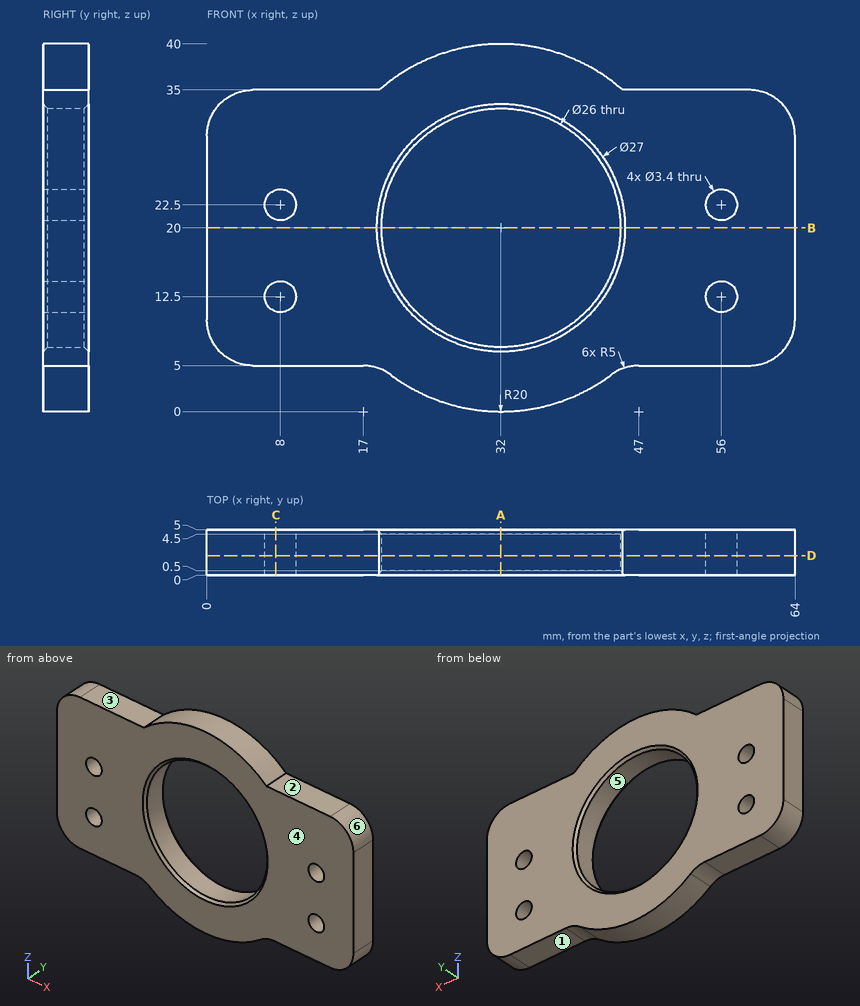
Input: dimensioned drawing with shaded views. Units: mm. Origin: part minimum x, y, z. A direction names the side the tool comes from. Round coordinates to 2 decimals unless told otherwise and drop trailing zeros. Loops run counter-clockwise (first coordinate to the right, second up) from the corner with the lowest first, then second, coordinate; pieces in that order, holes last. Notation, with made-up numbers: (67.5, 89.25) -> (85.5, 89.25) arc R20 cw to (85.5, 94.25) -> close; hole circle Ø10 at (-25, 84.5). An arc over 180 degrees is marked (long way). Answer as a JSON object with one key per item and string values. Group by question number.
Q1. Section query C-C (x = 7.5). Output: boundary loops of the cut face in (y, z).
Q2. Contact query for flat-ended pins moving along their axis: P1, Ø10, axis at x = 31, z = 12, coming from the +Y side; P2, Ø1.5, axis at y = 3.5, z = 14, coming from the -X side; P3, Ø1.5, axis at x = 51.5, y = 3.5, coming from the -Z side; P4, Ø1.5, axis at x = 13.5, y = 1.5, coming from the +Z side. Output: stop coordinate, or through.
Q3. Mould query, pull axis Z, two halves, no side actions, for the marked faces 4, 5 and 6. Classes: pulls with the +Z half, pulls with the -Z half, needs draft (parallel to the pull), parting line crosses it, or undercut.
Q4. Ray query, line 1 (Z direction, x = 56, y = 3.7); line 2 (Z direction, x = 32, y = 1.85); line 3 (X direction, y = 1.55, z = 14). Return the intervals inside material, ascending. Write a range as from..to.
Q5. Access query for the marked faces 1, 2 and 3. Directions: +Z, -Z, +X, -X, +Y, -Y. A direction counts if a zero-diameter tool reaches every point of the face in a straight line with its end or side. Return the directions, or none.
Q6. Section query A-A (x = 32). Output: boundary loops of the cut face in (y, z), plus the area to 3 significant figures.
Q7. Section query B-B (z = 20). Output: boundary loops of the cut face in (x, y), plus the area to 4 significant figures.
Q8. Section query D-D (y = 2.15). Output: boundary loops of the cut face in (x, z).
Completed:
{
 "1": {"outline": "(0, 5) -> (5, 5) -> (5, 10.88) -> (0, 10.88) -> close; (0, 14.12) -> (5, 14.12) -> (5, 20.88) -> (0, 20.88) -> close; (0, 24.12) -> (5, 24.12) -> (5, 35) -> (0, 35) -> close"},
 "2": {"P1": "y = 4.56", "P2": "x = 0", "P3": "z = 5", "P4": "z = 35"},
 "3": {"face 4": "needs draft", "face 5": "undercut", "face 6": "pulls with the +Z half"},
 "4": {"line 1": "5..10.8, 14.2..20.8, 24.2..35", "line 2": "0..7, 33..40", "line 3": "0..7.2, 8.8..20.47, 43.53..55.2, 56.8..64"},
 "5": {"face 1": "-Z, +X, +Y, -Y", "face 2": "+Z, +X, +Y, -Y", "face 3": "+Z, -X, +Y, -Y"},
 "6": {"outline": "(0, 0) -> (5, 0) -> (5, 6.5) -> (4.5, 7) -> (0.5, 7) -> (0, 6.5) -> close; (0, 33.5) -> (0.5, 33) -> (4.5, 33) -> (5, 33.5) -> (5, 40) -> (0, 40) -> close", "area": "69.5 mm²"},
 "7": {"outline": "(0, 0) -> (18.5, 0) -> (19, 0.5) -> (19, 4.5) -> (18.5, 5) -> (0, 5) -> close; (45, 0.5) -> (45.5, 0) -> (64, 0) -> (64, 5) -> (45.5, 5) -> (45, 4.5) -> close", "area": "189.5 mm²"},
 "8": {"outline": "(0, 10) arc R5 ccw to (5, 5) -> (17, 5) arc R5 cw to (20, 4) arc R20 ccw to (44, 4) arc R5 cw to (47, 5) -> (59, 5) arc R5 ccw to (64, 10) -> (64, 30) arc R5 ccw to (59, 35) -> (45.23, 35) arc R20 ccw to (18.77, 35) -> (5, 35) arc R5 ccw to (0, 30) -> close; hole circle Ø3.4 at (8, 12.5); hole circle Ø3.4 at (8, 22.5); hole circle Ø26 at (32, 20); hole circle Ø3.4 at (56, 12.5); hole circle Ø3.4 at (56, 22.5)"}
}
